```python
from build123d import *

# Parameters (mm, degrees)
SKETCH1_W           = 35
SKETCH1_H           = 35
BOSS_EXTRUDE1_DEPTH = 7.5
SKETCH2_W           = 24
SKETCH2_H           = 13
CUT_EXTRUDE2_DEPTH  = 5
SKETCH10_R          = 0.75
CUT_EXTRUDE7_DEPTH  = 7
SKETCH5_R           = 2.5
CUT_EXTRUDE11_DEPTH = 1
SKETCH11_R          = 2.25
CUT_EXTRUDE12_DEPTH = 5
CUT_EXTRUDE13_DEPTH = 10
CUT_EXTRUDE14_DEPTH = 10
CUT_EXTRUDE15_DEPTH = 4
BOSS_EXTRUDE2_DEPTH = 10
SKETCH17_R          = 3
CUT_EXTRUDE16_DEPTH = 1.5


with BuildPart() as part:
    # Sketch1 → Boss-Extrude1 (new body)
    with BuildSketch(Plane.XY):
        with Locations((-0.233740073, -3.509910016)):
            Rectangle(SKETCH1_W, SKETCH1_H)
    extrude(amount=BOSS_EXTRUDE1_DEPTH)

    # Sketch2 → Cut-Extrude2 (cut)
    with BuildSketch(Plane(origin=(0, 0, 0), x_dir=(-1, 0, 0), z_dir=(0, 0, -1))):
        with Locations((5.733740073, -3.509910016)):
            Rectangle(SKETCH2_W, SKETCH2_H)
    extrude(amount=-CUT_EXTRUDE2_DEPTH, mode=Mode.SUBTRACT)

    # Sketch10 → Cut-Extrude7 (cut)
    with BuildSketch(Plane(origin=(0, 13.990089984, 0), x_dir=(1, 0, 0), z_dir=(0, 1, 0))):
        with Locations((4.066259927, -3.75)):
            Circle(SKETCH10_R)
        with Locations((-1.933740073, -3.75)):
            Circle(SKETCH10_R)
    extrude(amount=-CUT_EXTRUDE7_DEPTH, mode=Mode.SUBTRACT)

    # Sketch5 → Cut-Extrude11 (cut)
    with BuildSketch(Plane.XY.offset(7.5)):
        with Locations((12.766259927, 0.490089984)):
            Circle(SKETCH5_R)
        with Locations((-4.233740073, -16.509910016)):
            Circle(SKETCH5_R)
    extrude(amount=-CUT_EXTRUDE11_DEPTH, mode=Mode.SUBTRACT)

    # Sketch11 → Cut-Extrude12 (cut)
    with BuildSketch(Plane.XY.offset(6.5)):
        with Locations((-4.233740073, -16.509910016)):
            Circle(SKETCH11_R)
        with Locations((12.766259927, 0.490089984)):
            Circle(SKETCH11_R)
    extrude(amount=-CUT_EXTRUDE12_DEPTH, mode=Mode.SUBTRACT)

    # Sketch13 → Cut-Extrude13 (cut)
    with BuildSketch(Plane.XZ.offset(21.009910016)):
        Polygon((9.766259927, 7.5), (12.766259927, 4.5), (15.766259927, 7.5), align=None)
    extrude(amount=-CUT_EXTRUDE13_DEPTH, mode=Mode.SUBTRACT)

    # Sketch15 → Cut-Extrude14 (cut)
    with BuildSketch(Plane(origin=(0, 13.990089984, 0), x_dir=(1, 0, 0), z_dir=(0, 1, 0))):
        Polygon((9.766259927, -7.5), (12.766259927, -4.5), (15.766259927, -7.5), align=None)
    extrude(amount=-CUT_EXTRUDE14_DEPTH, mode=Mode.SUBTRACT)

    # Sketch4 → Cut-Extrude15 (cut)
    with BuildSketch(Plane.XY.offset(7.5)):
        with BuildLine():
            Line((-11.233740073, -15.239910016), (-15.233740073, -15.239910016))
            ThreePointArc((-15.233740073, -15.239910016), (-16.503740073, -16.509910016), (-15.233740073, -17.779910016))
            Line((-15.233740073, -17.779910016), (-11.233740073, -17.779910016))
            ThreePointArc((-11.233740073, -17.779910016), (-9.963740073, -16.509910016), (-11.233740073, -15.239910016))
        make_face()
    extrude(amount=-CUT_EXTRUDE15_DEPTH, mode=Mode.SUBTRACT)

    # Sketch16 → Boss-Extrude2 (add)
    with BuildSketch(Plane(origin=(0, -11.009910016, 0), x_dir=(-1, 0, 0), z_dir=(0, -1, 0))):
        Polygon((-9.766259927, -7.5), (-15.766259927, -7.5), (-12.766259927, -4.5), align=None)
    extrude(amount=BOSS_EXTRUDE2_DEPTH)

    # Sketch17 → Cut-Extrude16 (cut)
    with BuildSketch(Plane.XY.offset(7.5)):
        with Locations((12.766259927, -16.509910016)):
            Circle(SKETCH17_R)
    extrude(amount=-CUT_EXTRUDE16_DEPTH, mode=Mode.SUBTRACT)


solid = part.part
```
Here's how the part is built. I have some questions about the finished solid (model axes, mm). A direction names the side the tool comes from. Give positions to 0.01 mm unless a question says otherwise; leave off trailing zeros. Loops run counter-clockwise (first coordinate to the right, second up) from the corner with the lowest first, then second, coordinate; pieces in that order, holes last. Notation, with made-up numbers: M 75,60 L 127,60 A34 ccw 127,99 Z; hole C 59,-2 d6. An arc over 180 degrees is marked long. Use one line per item in the form item = value. Start each with the question number.
Q1. Thinking about a two-plate mould opening in X: for faces 5 (the flat face through (-17.734, -3.8, 5.4)), 6 (the flat face through (7, -3, 0)), 7 (the flat face through (-2, 6.99, 4)), which applies, +X half, -X half, draft (parallel to the pull), parting line (faces both ways), or undercut?
Q2. Will these pins go through, and if not, where does the flat tip stop? pin 1 Ø4 at (x, y) = (12.77, 0.49) entering from +Z; pin 2 Ø2.5 at (y, z) = (-5.5, 3.5) entering from -X; pin 3 Ø0.9 at (x, z) = (11.5, 6.5) entering from +Y.
Q3. If we section it at D-D (y = -6.5): Write out the boundary of the cut face in (x, z), then the cut area to 4 significant figures.
Q4. Which directions (+Z, -Z, +X, -X, +Y, -Y) give clear straight access to the entire face, cutting with the end or side of a thin tool? Please do faces 1 (the flat face through (13, 1, 1.5)), 2 (the flat face through (11.245, 9.06, 6.021)), 3 (the flat face through (-6, 2.99, 2)), 4 (the cylindrical face through (3.471, 10.539, 4.206)).
Q5. I need wall thicknesses on line 1 along Y through (x, z) = (-8, 2); line 2 along Y through (x, z) = (-3.5, 4.75); line 3 along X through (y, z) = (-14.5, 7.25). Which ranges of each line are inside material? Lowest first, please.
Q6. If we section it at C-C (z = 0.5): Write out the boundary of the cut face in (x, y), then the cut area to 3 significant figures.
Q7. If we section it at B-B (x = -12): Write out the boundary of the cut face in (y, z).
Q8. If we section it at A-A (y = 8): Write out the boundary of the cut face in (x, z).
Taken from the geometry:
q1.face_5 = -X half
q1.face_6 = draft
q1.face_7 = undercut
q2.pin_1 = 1.5
q2.pin_2 = 6.27
q2.pin_3 = 3.99
q3.outline = M -17.73,5 L 6.27,5 L 6.27,0 L 17.27,0 L 17.27,7.5 L -17.73,7.5 Z
q3.area = 142.5 mm^2
q4.face_1 = +Z
q4.face_2 = +Z, +Y
q4.face_3 = -Z, -X
q4.face_4 = +Y
q5.line_1 = -21.01 to -10.01, 2.99 to 13.99
q5.line_2 = -21.01 to -18.64, -14.38 to -10.01, 2.99 to 13.99
q5.line_3 = -17.73 to -5.72, -2.75 to 10.54, 14.99 to 17.27
q6.outline = M -17.73,-21.01 L 17.27,-21.01 L 17.27,13.99 L -17.73,13.99 L -17.73,2.99 L 6.27,2.99 L 6.27,-10.01 L -17.73,-10.01 Z
q6.area = 913 mm^2
q7.outline = M -21.01,0 L -10.01,0 L -10.01,5 L 2.99,5 L 2.99,0 L 13.99,0 L 13.99,7.5 L -15.24,7.5 L -15.24,3.5 L -17.78,3.5 L -17.78,7.5 L -21.01,7.5 Z
q8.outline = M -17.73,0 L 17.27,0 L 17.27,7.5 L 15.77,7.5 L 12.77,4.5 L 9.77,7.5 L -17.73,7.5 Z; hole C -1.93,3.75 d1.5; hole C 4.07,3.75 d1.5
